```python
from build123d import *

# Parameters (mm, degrees)
F4_R = 5.99999


# Not quite as in the source:
# - a fillet or chamfer is up to 0.001 mm smaller than in the source, because OpenCascade refuses the exact size


with BuildPart() as f1:
    # F0 (on Front) → F1 (revolve)
    with BuildSketch(Plane.XZ):
        with BuildLine():
            Line((0, 31), (0, 0))
            Line((0, 0), (88, 0))
            Line((88, 0), (88, 15))
            Line((88, 15), (85, 15))
            Line((85, 15), (85, 20))
            Line((85, 20), (68, 20))
            Line((68, 20), (68, 31))
            Line((68, 31), (56, 31))
            ThreePointArc((56, 31), (50, 25), (44, 31))
            Line((44, 31), (0, 31))
        make_face()
    revolve(axis=Axis((44, 0, 0), (-1, 0, 0)))

    # F2 (on Front) → F3 (revolve, cut)
    with BuildSketch(Plane.XZ):
        Polygon((0, 25), (0, 0), (88, 0), (88, 6), (30, 6), (30, 16), (22, 16), (22, 20.5), (16.5, 20.5), (16.5, 12.5), (13.5, 12.5), (13.5, 16), (1.5, 16), (1.5, 25), align=None)
    revolve(axis=Axis((-10.2086656565, 0, 0), (-1, 0, 0)), mode=Mode.SUBTRACT)

    # F4 (radius 6 in the source; OpenCascade refuses exactly that, so slightly less here)
    f4_edges = [f1.edges().sort_by_distance(p)[0] for p in [
        (0, 0, -31),
    ]]
    fillet(f4_edges, radius=F4_R)


solid = f1.part
```
Build history of the part. All positions in model axes, mm. A direction names the side the tool comes from. Coordinates: 2 decimals unless noted, no trailing zeros. Order: outer loops, then holes, each group sorted by start corner. A loop starts at its lowest first (then second) coordinate and runs counter-clockwise, first axis right, second up.
Item 1: Saw through at B-B on x = 75. List the corners of the cut face in (y, z).
Filled in:
outline: circle Ø40 at (0, 0); hole circle Ø12 at (0, 0)
Item 2: Tool access for faces 4 (the cylindrical face through (61.916, 30.736, -4.036)), 5 (the cylindrical face through (19.212, -20.013, -4.444)), 6 (the cylindrical face through (86.479, 0.66, -14.985)), 7 (the flat face through (1.5, -16.3, 0.3)): list every direction of +Z, -Z, +X, -X, +Y, -Y with a clear straight run to the whole face (end or side of a thin tool).
Filled in:
face 4: +X, -X
face 5: none
face 6: +X
face 7: -X
Item 3: Saw through at A-A on x = 59.5. List the corners of the cut face in (y, z), then the cut area to 3 significant figures.
Filled in:
outline: circle Ø62 at (0, 0); hole circle Ø12 at (0, 0)
area: 2,910 mm2
Item 4: Mould opens along Y. For faces 1 (the cylindrical face through (24.734, 30.736, -4.036)), 2 (the cylindrical face through (59, 0, -6)), 3 (the flat face through (88, -6.5, 0.2)) say: released by +Y, released by -Y, zero draft, split by the parting line, or undercut.
Filled in:
face 1: split by the parting line
face 2: undercut
face 3: zero draft
Item 5: Drill centre lines: L1, parallel to X at y = 1, z = -14; L2, parallel to X at y = -14, z = -6; L3, parallel to Y at x = 9.5, z = 0. Where is each one in solid material? Low to high.
Filled in:
L1: x = 13.5 to 16.5, 30 to 88
L2: x = 13.5 to 16.5, 30 to 85
L3: y = -31 to -16, 16 to 31
Item 6: Drop flat-ended pins along their axis: pin 1 Ø1.5 at (x, y) = (55.5, -22.5) entering from +Z; pin 2 Ø6 at (x, y) = (17, -11.5) entering from +Z; pin 3 Ø2 at (x, y) = (40, 15.5) entering from -Z. Give the stop position or say it passes through.
Filled in:
pin 1: stops at z = 21.9
pin 2: stops at z = 29.81
pin 3: stops at z = -27.4
